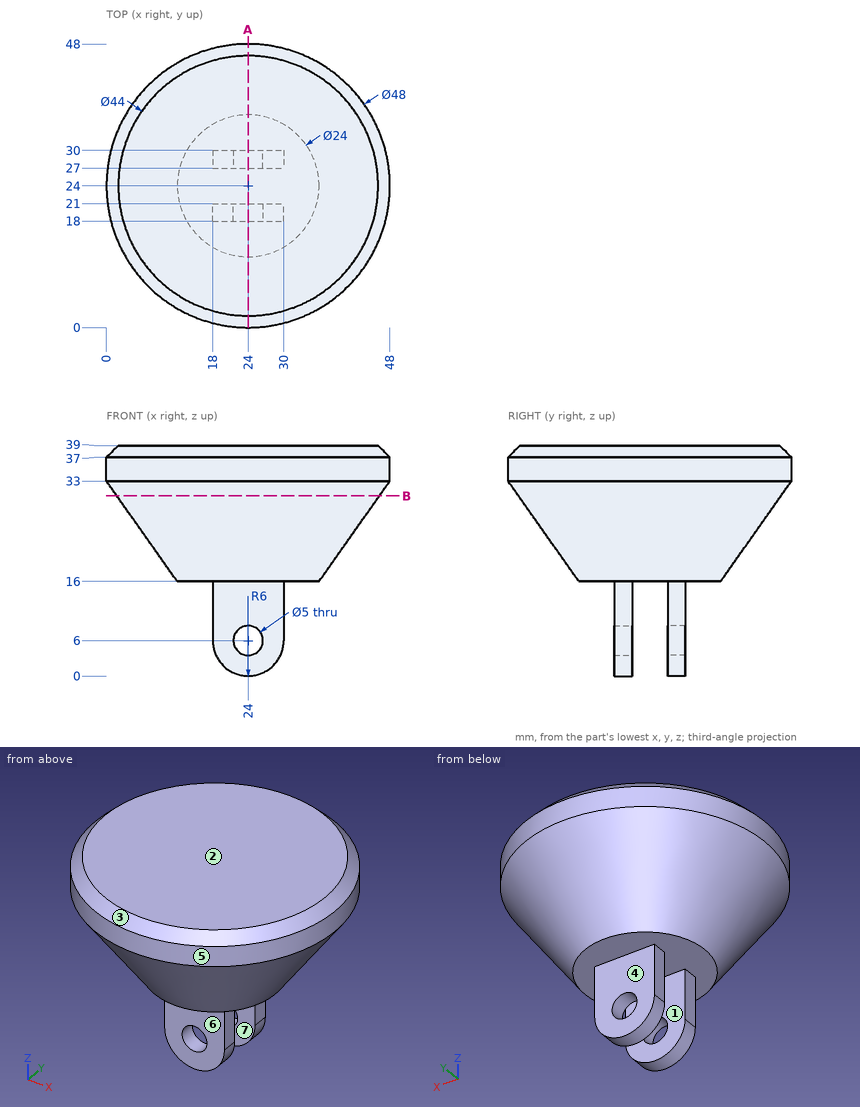
For this review, use the dimensioned drawing (mm, ordinates from the lowest corner) and the shaded views. A direction names the side the tool comes from. Round coordinates to 2 decimals unless told otherwise and drop trailing zeros. Write each loop counter-clockwise with the first axis right and the second up, starting at its lowest first coordinate (ties: lowest second). Pieces come first, ordered by that corner, then holes. Notation, with made-up numbers: (18.25, -22.75) -> (44.25, -22.75) arc R25 cw to (44.25, -8.75) -> close; hole circle Ø1 at (3.5, 87.25). An arc over 180 degrees is marked (long way). Answer in a Markdown table with one row per item.
Q1. Draft analysis for pull direction Y (two halves, no side actions). For the marked faces 1, 2, 3 and 4, state which applies: +Y half, -Y half, draft (parallel to the pull), parting line (faces both ways), or undercut.
The answers:
| item | result |
|---|---|
| face 1 | undercut |
| face 2 | draft |
| face 3 | parting line |
| face 4 | +Y half |
Q2. For the marked faces 5, 6 and 7, list the 3-axis set-ups (+Z, -Z, +X, -X, +Y, -Y) from which the entire face can be reached by the end or side of a thin tool; tool diameter is ignored.
The answers:
| item | result |
|---|---|
| face 5 | +Z, -Z |
| face 6 | -Z, +X, -X, -Y |
| face 7 | -Z, +X, -X |
Q3. Take a section at B-B, the plane z = 30.5. State the section outline as (x, y) points, then the cut area to 3 significant figures.
The answers:
| item | result |
|---|---|
| outline | circle Ø44.47 at (24, 24) |
| area | 1,550 mm² |
Q4. Take a section at A-A, the plane x = 24. State the section outline as (y, z) points.
The answers:
| item | result |
|---|---|
| outline | (0, 33) -> (12, 16) -> (18, 16) -> (18, 8.5) -> (21, 8.5) -> (21, 16) -> (27, 16) -> (27, 8.5) -> (30, 8.5) -> (30, 16) -> (36, 16) -> (48, 33) -> (48, 37) -> (46, 39) -> (2, 39) -> (0, 37) -> close; (18, 0) -> (21, 0) -> (21, 3.5) -> (18, 3.5) -> close; (27, 0) -> (30, 0) -> (30, 3.5) -> (27, 3.5) -> close |
Q5. To check wall thickness, follow L1, parallel to Y at x = 24.5, z = 9; L2, parallel to Z at x = 24, y = 29; L3, parallel to Z at x = 23, y = 26.5. State the ranges of each line that lie inside material, in increasing order. Write a range as [from, to].
The answers:
| item | result |
|---|---|
| L1 | [18, 21], [27, 30] |
| L2 | [0, 3.5], [8.5, 39] |
| L3 | [16, 39] |
Q6. Clearance check with flat-ended pins moving along their axes: pin 1 Ø10 at (x, z) = (34, 19.5) entering from -Y; pin 2 Ø3.5 at (y, z) = (28, 12) entering from +X; pin 3 Ø8 at (x, z) = (28.5, 24) entering from -Y. State where each tip first meets the part, or that it passes through.
The answers:
| item | result |
|---|---|
| pin 1 | y = 8.16 |
| pin 2 | x = 30 |
| pin 3 | y = 3.92 |
